Verification items for the finished model (mm, model axes). Face numbers are marked on the shaded views. A direction names the side the tool comes from. Round coordinates to 2 decimals unless told otherwise and drop trailing zeros. Write each loop counter-clockwise with the first axis right and the second up, starting at its lowest first coordinate (ties: lowest second). Pieces come first, ordered by that corner, then holes. Notation, with made-up numbers: (-28.75, 33) - (22.25, 33) arc R38 ccw to (22.25, 72) - close; hole circle Ø1 at (20.25, 60.5). An arc over 180 degrees is marked (long way). Answer as a JSON object with one key per item and string values.
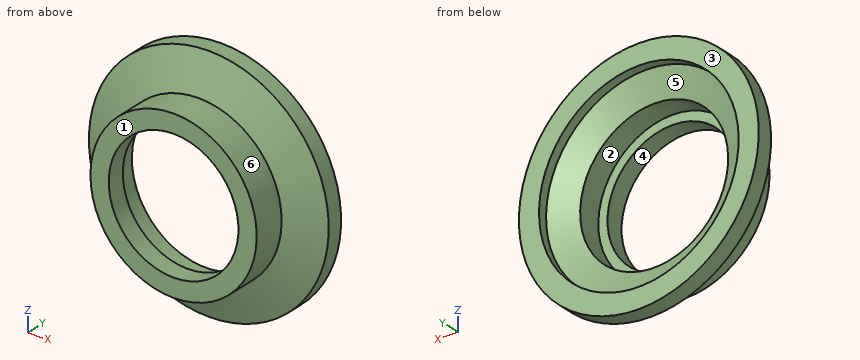
```python
from build123d import *

# Parameters (mm, degrees)
SKETCH3_R      = 4.6228
SKETCH3_R_2    = 4.1148
EXTRUDE2_DEPTH = 0.508
SKETCH6_R      = 4.1148
EXTRUDE5_DEPTH = 1.016
SKETCH10_R     = 3.6068
EXTRUDE7_DEPTH = 4.429


with BuildPart() as part:
    # Sketch1 → Revolve1 (revolve)
    with BuildSketch(Plane.XY, mode=Mode.PRIVATE) as revolve1_sk:
        Polygon((4.6228, 0), (4.6228, 2.303790062), (6.6675, 3.048), (6.6675, 3.937), (5.5499, 3.937), (5.5499, 3.429), (4.1148, 2.834562117), (4.1148, 0), align=None)
    revolve(revolve1_sk.sketch.rotate(Axis((0, 0, 0), (0, -1, 0)), 90), axis=Axis((0, 0, 0), (0, -1, 0)))  # turned: the seam where the file's is

    # Sketch3 → Extrude2 (cut)
    with BuildSketch(Plane.XZ):
        with Locations(Location((0, 0, 0), (0, 0, 90))):  # turned: the seam where the file's is
            Circle(SKETCH3_R)
        with Locations(Location((0, 0, 0), (0, 0, 90))):  # turned: the seam where the file's is
            Circle(SKETCH3_R_2, mode=Mode.SUBTRACT)
    extrude(amount=-EXTRUDE2_DEPTH, mode=Mode.SUBTRACT)

    # Sketch6 → Extrude5 (add)
    with BuildSketch(Plane.XZ.offset(-0.508)):
        with Locations(Location((0, 0, 0), (0, 0, 90))):  # turned: the seam where the file's is
            Circle(SKETCH6_R)
    extrude(amount=-EXTRUDE5_DEPTH)

    # Sketch10 → Extrude7 (cut, through all)
    with BuildSketch(Plane.XZ.offset(-0.508)):
        with Locations(Location((0, 0, 0), (0, 0, 270))):  # turned: the seam where the file's is
            Circle(SKETCH10_R)
    extrude(amount=-EXTRUDE7_DEPTH, mode=Mode.SUBTRACT)


solid = part.part
```
Q1. Section check C-C, the plane y = 1.35. Record the cut outline in (x, z), then the cut area to 3 significant figures.
Geometry check:
{"outline": "circle Ø9.25 at (0, 0); hole circle Ø7.21 at (0, 0)", "area": "26.3 mm2"}
Q2. Set-up check for the marked faces 1 and 2: record each of +Z, -Z, +X, -X, +Y, -Y from which the full face is reachable in a straight line by a thin tool's end or side.
Geometry check:
{"face 1": "+Z, -Z, +X, -X, -Y", "face 2": "+Y"}
Q3. Gauge pin test, flat end, axial feed: P1, Ø2, axis at x = 4.5, y = 1.5, coming from the +Z side. Record the tip position at first contact, or that the pin passes through.
Geometry check:
{"P1": "stops at z = 3.02"}
Q4. Release check for a two-part mould opening along X. For the marked faces 3, 4, 5 and 6 record: released by +X, released by -X, zero draft, split by the parting line, or undercut.
Geometry check:
{"face 3": "zero draft", "face 4": "undercut", "face 5": "undercut", "face 6": "split by the parting line"}
Q5. Section check A-A, the plane x = 0. Record the cut outline in (y, z).
Geometry check:
{"outline": "(0.51, -4.62) - (2.3, -4.62) - (3.05, -6.67) - (3.94, -6.67) - (3.94, -5.55) - (3.43, -5.55) - (2.83, -4.11) - (1.52, -4.11) - (1.52, -3.61) - (0.51, -3.61) - close; (0.51, 3.61) - (1.52, 3.61) - (1.52, 4.11) - (2.83, 4.11) - (3.43, 5.55) - (3.94, 5.55) - (3.94, 6.67) - (3.05, 6.67) - (2.3, 4.62) - (0.51, 4.62) - close"}
Q6. Material ranges on line 1 along X through (y, z) = (0.95, 0); line 2 along X through (y, z) = (3.8, 0); line 3 along Z through (x, y) = (-0.5, 1.95), recorded low to high. Write a range as [from, to].
Geometry check:
{"line 1": "x = [-4.62, -3.61], [3.61, 4.62]", "line 2": "x = [-6.67, -5.55], [5.55, 6.67]", "line 3": "z = [-4.6, -4.08], [4.08, 4.6]"}
Q7. Section check D-D, the plane y = 2.6. Record the cut outline in (x, z).
Geometry check:
{"outline": "circle Ø10.87 at (0, 0); hole circle Ø8.23 at (0, 0)"}
Q8. Section check B-B, the plane z = 0. Record the cut outline in (x, y), then the cut area to 3 significant figures.
Geometry check:
{"outline": "(-6.67, 3.05) - (-4.62, 2.3) - (-4.62, 0.51) - (-3.61, 0.51) - (-3.61, 1.52) - (-4.11, 1.52) - (-4.11, 2.83) - (-5.55, 3.43) - (-5.55, 3.94) - (-6.67, 3.94) - close; (3.61, 0.51) - (4.62, 0.51) - (4.62, 2.3) - (6.67, 3.05) - (6.67, 3.94) - (5.55, 3.94) - (5.55, 3.43) - (4.11, 2.83) - (4.11, 1.52) - (3.61, 1.52) - close", "area": "7.36 mm2"}
